```python
from build123d import *

# Parameters (mm, degrees)
SKETCH1_W           = 5.3528
SKETCH1_H           = 5.3528
SKETCH1_W_2         = 3.3528
SKETCH1_H_2         = 3.3528
BOSS_EXTRUDE1_DEPTH = 9.525
BOSS_EXTRUDE2_START = -5.3528
BOSS_EXTRUDE2_DEPTH = 5.3528


with BuildPart() as part:
    # Sketch1 → Boss-Extrude1 (new, symmetric)
    with BuildSketch(Plane(origin=(0, 0, 0), x_dir=(0, 0, -1), z_dir=(1, 0, 0))):
        with Locations((16.646784182, 0)):
            Rectangle(SKETCH1_W, SKETCH1_H)
        with Locations((16.646784182, 0)):
            Rectangle(SKETCH1_W_2, SKETCH1_H_2, mode=Mode.SUBTRACT)
    extrude(amount=BOSS_EXTRUDE1_DEPTH, both=True)

    # Sketch2 → Boss-Extrude2 (add)
    with BuildSketch(Plane.XZ.offset(2.6764).offset(BOSS_EXTRUDE2_START)):
        with BuildLine():
            Line((-9.525, -13.970384182), (-9.525, -10.258084471))
            ThreePointArc((-9.525, -10.258084471), (0, -6.087615818), (9.525, -10.258084471))
            Line((9.525, -10.258084471), (9.525, -13.970384182))
            Line((9.525, -13.970384182), (-9.525, -13.970384182))
        make_face()
    extrude(amount=BOSS_EXTRUDE2_DEPTH)

    # Sketch3 → Cut-Revolve1 (revolve, cut)
    with BuildSketch(Plane(origin=(0, 0, 0), x_dir=(1, 0, 0), z_dir=(0, 1, 0))):
        with BuildLine():
            Line((-9.525, 10.258084471), (-9.525, -8.791915529))
            Line((-9.525, -8.791915529), (9.525, -8.791915529))
            Line((9.525, -8.791915529), (9.525, 10.258084471))
            ThreePointArc((9.525, 10.258084471), (0, 6.087615818), (-9.525, 10.258084471))
        make_face()
    revolve(axis=Axis((9.525, 0, -19.323184182), (-1, 0, 0)), mode=Mode.SUBTRACT)


solid = part.part
```
Geometry: final body of the model. Coordinates: model frame, mm. A direction names the side the tool comes from. Coordinates: 2 decimals unless noted, no trailing zeros. Order: outer loops, then holes, each group sorted by start corner. A loop starts at its lowest first (then second) coordinate and runs counter-clockwise, first axis right, second up.
Item 1: Draft query along Z for faces 3 (the face through (0, 0, -19.323)), 4 (the face through (0, 1.676, -17)), 5 (the face through (0, -2.676, -13)). Return one class per face: released by +Z, released by -Z, zero draft, split by the parting line, or undercut.
Answer:
face 3: released by -Z
face 4: undercut
face 5: zero draft
Item 2: Section query A-A (z = -17.5). Output: boundary loops of the cut face in (x, y) (3 decimals), then the cut area to 3 significant figures.
Answer:
outline: (-9.525, -2.676) - (9.525, -2.676) - (9.525, -1.676) - (-9.525, -1.676) - close; (-9.525, 1.676) - (9.525, 1.676) - (9.525, 2.676) - (-9.525, 2.676) - close
area: 38.1 mm2
Item 3: Material intervals for line 1 along Y through (x, z) = (2, -17); line 2 along Z through (x, y) = (4, 0.4); line 3 along Z through (x, y) = (4.25, -0.6), sorted ascending.
Answer:
line 1: y = -2.68 to -1.68, 1.68 to 2.68
line 2: z = -19.32 to -18.32, -14.97 to -6.73
line 3: z = -19.32 to -18.32, -14.97 to -6.82
Item 4: Contact query for flat-ended pins moving along their axis: P1, Ø1, axis at x = -1, y = 1.5, coming from the +Z side; P2, Ø1, axis at x = 1, y = -0.5, coming from the +Z side. Output: stop coordinate, or through.
Answer:
P1: stops at z = -6.15
P2: stops at z = -6.1
Item 5: Access query for faces 1 (the face through (0, 0, -18.323)), 2 (the face through (0, 2.676, -13)). Directions: +Z, -Z, +X, -X, +Y, -Y. A direction counts if a zero-diameter tool reaches every point of the face in a straight line with its end or side. Return the directions, or none.
Answer:
face 1: +X, -X
face 2: +Z, -Z, +X, -X, +Y
